The drawing under review shows one solid part. Ordinate dimensions are in mm from its lowest x, y, z. Round coordinates to 2 decimals unless told otherwise and drop trailing zeros. Order: outer loops, then holes, each group sorted by start corner. A loop starts at its lowest first (then second) coordinate and runs counter-clockwise, first axis right, second up.
1) Clearance check with flat-ended pins moving along their axes: P1, Ø2, axis at y = 86, z = 3.5, coming from the -X side; P2, Ø2, axis at y = 56.5, z = 9.5, coming from the -X side; P3, Ø10.5, axis at x = 173.5, y = 191.8, coming from the +Z side; P4, Ø6, axis at y = 114.5, z = 14.5, coming from the -X side. State where each tip first meets the part, or that it passes through.
2) Consider section A-A (y = 148.5). Give the boundary of the cut face in (x, z).
3) Consider section D-D (x = 270.5). Give the boundary of the cut face in (y, z) (1 decimal).
4) To check wall thickness, follow L1, parallel to Y at x = 207.5, z = 1.75 (1 decimal); L2, parallel to Y at x = 148.5, z = 5.5; L3, parallel to Y at x = 123.5, z = 7.5. State the ranges of each line that lie inside material, in increasing order.
5) Consider section C-C (y = 216). Give the boundary of the cut face in (x, z).
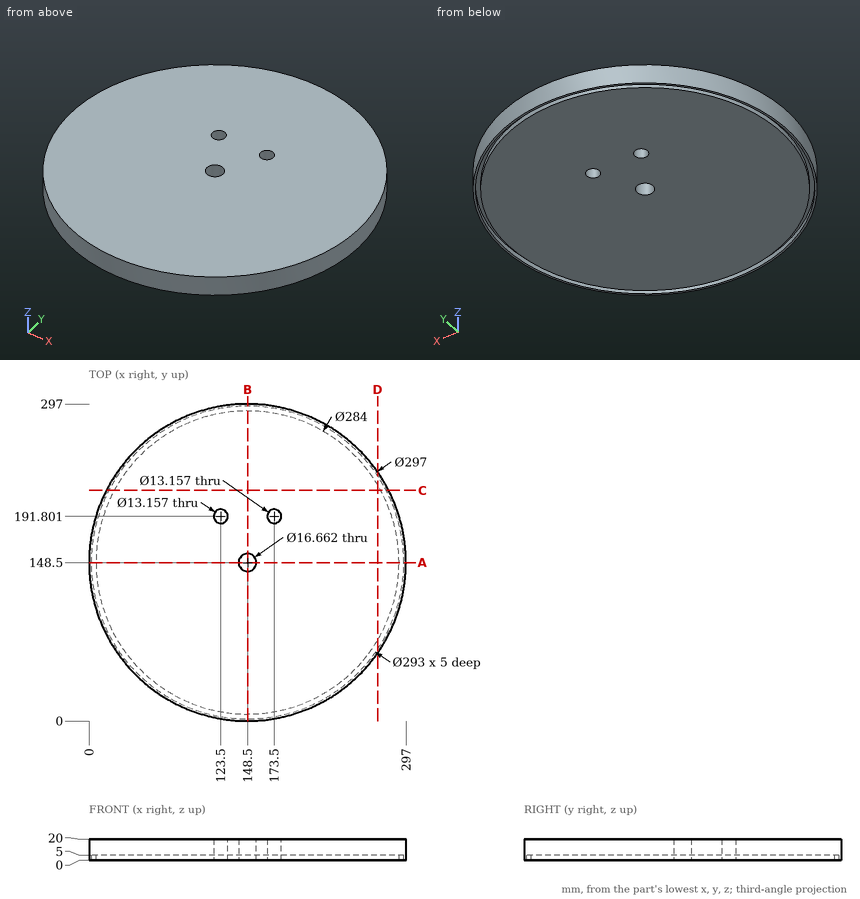
Answer below:
1. P1: stops at x = 13.33
1. P2: stops at x = 31.15
1. P3: passes through
1. P4: stops at x = 3.27
2. outline: (0, 0) - (2, 0) - (2, 5) - (6.5, 5) - (6.5, 0) - (140.17, 0) - (140.17, 20) - (0, 20) - close; (156.83, 0) - (290.5, 0) - (290.5, 5) - (295, 5) - (295, 0) - (297, 0) - (297, 20) - (156.83, 20) - close
3. outline: (63.8, 0) - (67.4, 0) - (67.4, 5) - (75.8, 5) - (75.8, 0) - (221.2, 0) - (221.2, 5) - (229.6, 5) - (229.6, 0) - (233.2, 0) - (233.2, 20) - (63.8, 20) - close
4. L1: y = 12.2 to 14.4, 19.3 to 277.7, 282.6 to 284.8
4. L2: y = 0 to 140.17, 156.83 to 297
4. L3: y = 2.12 to 185.22, 198.38 to 294.88
5. outline: (16.23, 0) - (18.48, 0) - (18.48, 5) - (23.57, 5) - (23.57, 0) - (273.43, 0) - (273.43, 5) - (278.52, 5) - (278.52, 0) - (280.77, 0) - (280.77, 20) - (16.23, 20) - close
